Model file for the job. Use its own axes, mm. A direction names the side the tool comes from. Give positions to 0.01 mm unless a question says otherwise; leave off trailing zeros. Loops run counter-clockwise (first coordinate to the right, second up) from the corner with the lowest first, then second, coordinate; pieces in that order, holes last. Notation, with made-up numbers: M -13.5,79.5 L 27.5,79.5 A23 ccw 27.5,100.5 Z; hole C 50.5,1 d5. An arc over 180 degrees is marked long. Answer in a Markdown table with one row per item.
Autodesk Inventor part; units mm, degrees
ref_plane "YZ Plane" through (0, 0, 0) normal (1, 0, 0) x (0, 1, 0)
ref_plane "XZ Plane" through (0, 0, 0) normal (0, 1, 0) x (-1, 0, 0)
ref_plane "XY Plane" through (0, 0, 0) normal (0, 0, 1) x (1, 0, 0)
sketch "スケッチ1" plane through (0, 0, 0) normal (0, 0, 1) x (1, 0, 0)
  line L0 (10, -10) -> (-10, -10) construction
  line L1 (-10, -10) -> (-10, 10) construction
  line L2 (-10, 10) -> (10, 10) construction
  line L3 (10, 10) -> (10, -10) construction
  line L4 (10, -10) -> (-10, 10) construction
  line L5 (-10, -10) -> (10, 10) construction
  line L6 (12.5, -12.5) -> (-12.5, -12.5) construction
  line L7 (-12.5, -12.5) -> (-12.5, 12.5) construction
  line L8 (-12.5, 12.5) -> (12.5, 12.5) construction
  line L9 (12.5, 12.5) -> (12.5, -12.5) construction
  line L10 (12.5, -12.5) -> (-12.5, 12.5) construction
  line L11 (-12.5, -12.5) -> (12.5, 12.5) construction
  circle A0 centre (10, 10) radius 1.25
  circle A1 centre (-10, 10) radius 1.25
  circle A2 centre (10, -10) radius 1.25
  circle A3 centre (-10, -10) radius 1.25
  circle A4 centre (20, 20) radius 1.75
  line L12 (20, -20) -> (-20, -20) construction
  line L13 (-20, -20) -> (-20, 20) construction
  line L14 (-20, 20) -> (20, 20) construction
  line L15 (20, 20) -> (20, -20) construction
  line L16 (20, -20) -> (-20, 20) construction
  line L17 (-20, -20) -> (20, 20) construction
  circle A5 centre (-20, 20) radius 1.6
  circle A6 centre (20, -20) radius 1.75
  circle A7 centre (-20, -20) radius 1.75
  arc A8 (21.7678, 18.2322) -> (17.5, 20) centre (20, 20) ccw
  line L18 (17.5, 20) -> (17.5, 20)
  line L19 (13, 15.5) -> (-13, 15.5)
  circle A9 centre (0, 0) radius 11.3921
  arc A10 (13, 15.5) -> (17.5, 20) centre (13, 20) ccw
  line L20 (21.7678, 18.2322) -> (15.5637, 12.0282)
  line L21 (14.3921, 9.1997) -> (14.3921, -9.1997)
  arc A11 (15.5637, 12.0282) -> (14.3921, 9.1997) centre (18.3921, 9.1997) ccw
  line L22 (20, 0) -> (-20, 0) construction
  line L23 (0, 20) -> (0, -20) construction
  arc A12 (17.5, -20) -> (21.7678, -18.2322) centre (20, -20) ccw
  line L24 (17.5, -20) -> (17.5, -20)
  line L25 (13, -15.5) -> (-13, -15.5)
  arc A13 (17.5, -20) -> (13, -15.5) centre (13, -20) ccw
  line L26 (21.7678, -18.2322) -> (15.5637, -12.0282)
  arc A14 (14.3921, -9.1997) -> (15.5637, -12.0282) centre (18.3921, -9.1997) ccw
  circle A15 centre (10, 10) radius 2.75 construction
  arc A16 (-17.5, 20) -> (-21.7678, 18.2322) centre (-20, 20) ccw
  arc A17 (-17.5, 20) -> (-13, 15.5) centre (-13, 20) ccw
  line L27 (-21.7678, 18.2322) -> (-15.5637, 12.0282)
  line L28 (-14.3921, 9.1997) -> (-14.3921, -9.1997)
  arc A18 (-14.3921, 9.1997) -> (-15.5637, 12.0282) centre (-18.3921, 9.1997) ccw
  arc A19 (-15.5637, -12.0282) -> (-14.3921, -9.1997) centre (-18.3921, -9.1997) ccw
  line L29 (-21.7678, -18.2322) -> (-15.5637, -12.0282)
  arc A20 (-21.7678, -18.2322) -> (-17.5, -20) centre (-20, -20) ccw
  line L30 (-17.5, -20) -> (-17.5, -20)
  arc A21 (-13, -15.5) -> (-17.5, -20) centre (-13, -20) ccw
  line L31 (-17.5, 20) -> (-17.5, 20)
  dimension "d0" = 20
  dimension "d1" = 20
  dimension "d2" = 25
  dimension "d3" = 25
  dimension "d4" = 2.5
  dimension "d5" = 2.5
  dimension "d6" = 2.5
  dimension "d7" = 2.5
  dimension "d8" = 3.5
  dimension "d9" = 40
  dimension "d10" = 40
  dimension "d11" = 3.2
  dimension "d12" = 3.5
  dimension "d13" = 3.5
  dimension "d14" = 2.5
  dimension "d18" = 4
  dimension "d19" = 3
  dimension "d20" = 45
  dimension "d21" = 5.5
  dimension "d22" = 3
extrude "押し出し1" add sketch "スケッチ1" along normal blind 3
equation "\"d1\" = d0"
equation "\"d3\" = d2"
equation "\"d5\" = d4"
equation "\"d6\" = d4"
equation "\"d7\" = d4"
equation "\"d22\" = d19"
properties part number "Fan_support_stand"
(1) Saw through at D-D, the plane y = -10. Give the cut face in (x, z).
Established:
| item | result |
|---|---|
| outline | M -14.47,0 L -11.25,0 L -11.25,3 L -14.47,3 Z; M -8.75,0 L -5.46,0 L -5.46,3 L -8.75,3 Z; M 5.46,0 L 8.75,0 L 8.75,3 L 5.46,3 Z; M 11.25,0 L 14.47,0 L 14.47,3 L 11.25,3 Z |
(2) Flat gauge pins, fed straight in: P1, Ø4.5, axis at x = -20, y = -20, coming from the +Z side; P2, Ø1.5, axis at y = 1.5, z = 2, coming from the -X side; P3, Ø1.5, axis at x = -2.5, z = 1, coming from the -Y side; P4, Ø0.9, axis at x = 3.5, z = 1, coming from the +Y side. Where does each tip first touch, or does it go through?
Established:
| item | result |
|---|---|
| P1 | stops at z = 3 |
| P2 | stops at x = -14.39 |
| P3 | stops at y = -15.5 |
| P4 | stops at y = 15.5 |
(3) Saw through at B-B, the plane x = 0. Give the cut face in (y, z), and give its area (3 significant figures).
Established:
| item | result |
|---|---|
| outline | M -15.5,0 L -11.39,0 L -11.39,3 L -15.5,3 Z; M 11.39,0 L 15.5,0 L 15.5,3 L 11.39,3 Z |
| area | 24.6 mm2 |
(4) Wall check: L1, parallel to Y at x = 0, z = 1.9; L2, parallel to Y at x = -20, z = 2; L3, parallel to Y at x = -12.5, z = 1.8. Give the ranges that are in metal, low to high.
Established:
| item | result |
|---|---|
| L1 | y = -15.5 to -11.39, 11.39 to 15.5 |
| L2 | y = -22.5 to -21.75, -18.25 to -16.46, 16.46 to 18.4, 21.6 to 22.5 |
| L3 | y = -15.5 to 15.5 |
(5) Which spindle directions (+Z, -Z, +X, -X, +Y, -Y) get a long thin tool onto all of the face, cutting with end or side? Do faces 1 (the cylindrical face through (-16.147, 16.783, 1.479)), 2 (the flat face through (-18.709, -15.174, 1.479)), 3 (the flat face through (0, 12, 3)), 4 (the flat face through (0, 12, 0)), 5 (the cylindrical face through (14.705, -10.751, 1.479)). Say none if no direction does.
Established:
| item | result |
|---|---|
| face 1 | +Z, -Z, +Y |
| face 2 | +Z, -Z, -X |
| face 3 | +Z, +X, -X, +Y, -Y |
| face 4 | -Z, +X, -X, +Y, -Y |
| face 5 | +Z, -Z, +X |
(6) Saw through at A-A, the plane y = 0. Give the cut face in (x, z), and give its area (3 significant figures).
Established:
| item | result |
|---|---|
| outline | M -14.39,0 L -11.39,0 L -11.39,3 L -14.39,3 Z; M 11.39,0 L 14.39,0 L 14.39,3 L 11.39,3 Z |
| area | 18.0 mm2 |
(7) Saw through at C-C, the plane z = 0.55. Count the separate pieces of the cut face and the enclosed holes in it, and give its area (3 significant figures).
Established:
| item | result |
|---|---|
| separate pieces | 1 |
| enclosed holes | 9 |
| area | 595 mm2 |
(8) Mould opens along Y. For faces 6 (the cylindrical face through (16.217, 16.853, 1.479)), 7 (the cylindrical face through (16.147, -16.783, 1.479)), 8 (the flat face through (-18.709, 15.174, 1.479)) say: pulls with the +Y half, pulls with the -Y half, needs draft (parallel to the pull), parting line crosses it, or undercut.
Established:
| item | result |
|---|---|
| face 6 | pulls with the +Y half |
| face 7 | pulls with the -Y half |
| face 8 | undercut |
